Verification items for the finished model (mm, model axes). Coordinates: 2 decimals unless noted, no trailing zeros. Order: outer loops, then holes, each group sorted by start corner. A loop starts at its lowest first (then second) coordinate and runs counter-clockwise, first axis right, second up. Notation, with made-up numbers: M 13.25,57.5 L 51.25,57.5 A26 ccw 51.25,89.5 Z; hole C 15.25,-18 d11. An arc over 180 degrees is marked long. Return JSON: item names as keys, results as strings.
```python
from build123d import *

# Parameters (mm, degrees)
F0_R     = 9
F0_R_2   = 7
F1_DEPTH = 415
F5_R     = 11
F5_R_2   = 7
F6_DEPTH = 330
F7_R     = 7
F8_DEPTH = 422.245019476


with BuildPart() as f1:
    # F0 (on Right) → F1 (new body)
    with BuildSketch(Plane.YZ):
        Circle(F0_R)
        Circle(F0_R_2, mode=Mode.SUBTRACT)
    extrude(amount=F1_DEPTH)

    # F5 (on offset) → F6 (join)
    with BuildSketch(Plane(origin=(-1.3846092047, -3.8041825246, 0), x_dir=(-0.9396926208, 0.3420201433, 0), z_dir=(0.3420201433, 0.9396926208, 0))):
        with Locations((-46.9846310393, 19)):
            Circle(F5_R)
        with Locations((-46.9846310393, 19)):
            Circle(F5_R_2, mode=Mode.SUBTRACT)
    extrude(amount=F6_DEPTH)

    # F7 (on face) → F8 (cut, through all)
    with BuildSketch(Plane(origin=(-1.3846092047, -3.8041825246, 0), x_dir=(0.9396926208, -0.3420201433, 0), z_dir=(-0.3420201433, -0.9396926208, 0))):
        with Locations((46.9846310393, 19)):
            Circle(F7_R)
    extrude(amount=-F8_DEPTH, mode=Mode.SUBTRACT)


solid = f1.part
```
Q1. Material ranges on line 1 along Z through (x, y) = (162, 0); line 2 along Y through (x, z) = (311, 4.5); line 3 along Y through (x, z) = (385.5, -5), recorded low to high.
Values:
{"line 1": "-9 to -7, 7 to 9", "line 2": "-7.79 to -5.36, 5.36 to 7.79", "line 3": "-7.48 to -4.9, 4.9 to 7.48"}
Q2. Draft check along Z on faces 1 (the face through (204.595, 6.466, -2.681)), 2 (the face through (155.78, 290.17, 11.82)). Enter one of: pulls with the +Z half, pulls with the -Z half, needs draft (parallel to the pull), parting line crosses it, or undercut.
Values:
{"face 1": "undercut", "face 2": "needs draft"}
Q3. Cross-section at B-B, the plane x = 229.5. Record the boundary of the cut face in (y, z).
Values:
{"outline": "C 0,0 d18; hole C 0,0 d14"}
Q4. Cross-section at A-A, the plane z = 0. Record the boundary of the cut face in (x, y), and give its area (3 significant figures).
Values:
{"outline": "M 0,-9 L 415,-9 L 415,-7 L 0,-7 Z; M 0,7 L 415,7 L 415,9 L 0,9 Z", "area": "1,660 mm^2"}
Q5. Go/stop test with flat-tipped pins: pin 1 (1 mm diameter, centred on x = 339, z = 1.5, fed in from +Y); pin 2 (8 mm diameter, centred on y = 237.5, z = 18, fed in from +X). Record where each tip stops, or that it passes through.
Values:
{"pin 1": "y = 8.94", "pin 2": "x = 149.58"}
